Part model, mm, in its own coordinate system. A direction names the side the tool comes from. Round coordinates to 2 decimals unless told otherwise and drop trailing zeros. Write each loop counter-clockwise with the first axis right and the second up, starting at its lowest first coordinate (ties: lowest second). Pieces come first, ordered by that corner, then holes. Notation, with made-up numbers: (76, 26.5) -> (111, 26.5) arc R20 cw to (111, 45.5) -> close; hole circle Ø9 at (49.5, 82). An arc over 180 degrees is marked (long way). Return JSON: item names as keys, results as strings. Group by question number.
(1) Tool access for faces 1 (the flat face through (4, 4, -7)), 2 (the flat face through (32, 15, -6)), 3 (the cylindrical face through (1.829, 28.145, -4.098)): list every direction of +Z, -Z, +X, -X, +Y, -Y with a clear straight run to the whole face (end or side of a thin tool).
(2) Drill centre lines: L1, parallel to Y at x = 62.25, z = -8.45; L2, parallel to Y at x = 62.25, z = -4.25; L3, parallel to X at y = 2.7, z = -3.25. Where is each one in solid material? Low to high. Write a range as from..to.
(3) Saw through at B-B (y = 15). List the corners of the cut face in (x, z).
(4) Saw through at C-C (z = -8.25). List the corners of the cut face in (x, y).
(5) Saw through at A-A (z = -1.5). List the corners of the cut face in (x, y), plus the area to 3 significant figures.
(6) Saw through at D-D (x = 27). List the corners of the cut face in (y, z), plus the area to 3 significant figures.
(7) Mould opens along Y. For faces 4 (the cylindrical face through (0.9, 29.14, -4.56)), 5 (the cylindrical face through (63.405, 2.221, -3.253)), 6 (the cylindrical face through (2.49, 29.283, -8.014)), 7 (the cylindrical face through (-5.5, 15.1, -7.5)) say: +Y half, -Y half, draft (parallel to the pull), parting line (faces both ways), or undercut.
(8) Drop flat-ended pins along their axis: pin 1 Ø3 at (x, y) = (62.25, 27.3) entering from -Z; pin 2 Ø2 at (y, z) = (10, -3.5) entering from -X; pin 3 Ø0.7 at (y, z) = (20.5, 0.5) entering from -X. Give the stop position or say it passes through.
from build123d import *

# Parameters (mm, degrees)
PAD002_DEPTH    = 9
POCKET002_DEPTH = 6
PAD003_DEPTH    = 0.6
SKETCH007_R     = 2
POCKET003_DEPTH = 2
SKETCH008_R     = 1.25
POCKET004_DEPTH = 10
PAD004_DEPTH    = 3


with BuildPart() as part:
    # Sketch004 → Pad002 (new body)
    with BuildSketch(Plane.XY):
        with BuildLine():
            Line((0, 27), (0, 3))
            ThreePointArc((0, 3), (0.87868, 0.87868), (3, 0))
            Line((3, 0), (62, 0))
            ThreePointArc((62, 0), (64.12132, 0.87868), (65, 3))
            Line((65, 3), (65, 27))
            ThreePointArc((65, 27), (64.12132, 29.12132), (62, 30))
            Line((62, 30), (3, 30))
            ThreePointArc((3, 30), (0.87868, 29.12132), (0, 27))
        make_face()
    extrude(amount=PAD002_DEPTH)

    # Sketch005 → Pocket002 (cut)
    with BuildSketch(Plane.XY.offset(9)):
        with BuildLine():
            Line((1.6, 27), (1.6, 3))
            ThreePointArc((1.6, 3), (2.010051, 2.010051), (3, 1.6))
            Line((3, 1.6), (62, 1.6))
            ThreePointArc((62, 1.6), (62.989949, 2.010051), (63.4, 3))
            Line((63.4, 3), (63.4, 27))
            ThreePointArc((63.4, 27), (62.989949, 27.989949), (62, 28.4))
            Line((62, 28.4), (3, 28.4))
            ThreePointArc((3, 28.4), (2.010051, 27.989949), (1.6, 27))
        make_face()
    extrude(amount=-POCKET002_DEPTH, mode=Mode.SUBTRACT)

    # Sketch006 → Pad003 (join)
    with BuildSketch(Plane.XY.offset(9)):
        with BuildLine():
            Line((1.1, 27), (1.1, 3))
            ThreePointArc((1.1, 3), (1.656497, 1.656497), (3, 1.1))
            Line((3, 1.1), (62, 1.1))
            ThreePointArc((62, 1.1), (63.343503, 1.656497), (63.9, 3))
            Line((63.9, 3), (63.9, 27))
            ThreePointArc((63.9, 27), (63.343503, 28.343503), (62, 28.9))
            Line((62, 28.9), (3, 28.9))
            ThreePointArc((3, 28.9), (1.656497, 28.343503), (1.1, 27))
        make_face()
        with BuildLine():
            Line((1.6, 27), (1.6, 3))
            ThreePointArc((1.6, 3), (2.010051, 2.010051), (3, 1.6))
            Line((3, 1.6), (62, 1.6))
            ThreePointArc((62, 1.6), (62.989949, 2.010051), (63.4, 3))
            Line((63.4, 3), (63.4, 27))
            ThreePointArc((63.4, 27), (62.989949, 27.989949), (62, 28.4))
            Line((62, 28.4), (3, 28.4))
            ThreePointArc((3, 28.4), (2.010051, 27.989949), (1.6, 27))
        make_face(mode=Mode.SUBTRACT)
    extrude(amount=PAD003_DEPTH)

    # Sketch007 → Pocket003 (cut)
    with BuildSketch(Plane.XY):
        with Locations((2.75, 27.3)):
            Circle(SKETCH007_R)
        with Locations((62.25, 27.3)):
            Circle(SKETCH007_R)
        with Locations((62.25, 2.7)):
            Circle(SKETCH007_R)
        with Locations((2.75, 2.7)):
            Circle(SKETCH007_R)
    extrude(amount=POCKET003_DEPTH, mode=Mode.SUBTRACT)

    # Sketch008 → Pocket004 (cut)
    with BuildSketch(Plane.XY):
        with Locations((2.75, 27.3)):
            Circle(SKETCH008_R)
        with Locations((62.25, 27.3)):
            Circle(SKETCH008_R)
        with Locations((2.75, 2.7)):
            Circle(SKETCH008_R)
        with Locations((62.25, 2.7)):
            Circle(SKETCH008_R)
    extrude(amount=POCKET004_DEPTH, mode=Mode.SUBTRACT)

    # Sketch009 → Pad004 (join)
    with BuildSketch(Plane.XY):
        with BuildLine():
            ThreePointArc((0, 20.5), (-5.5, 15), (0, 9.5))
            Line((0, 11.5), (0, 9.5))
            ThreePointArc((0, 18.5), (-3.5, 15), (0, 11.5))
            Line((0, 20.5), (0, 18.5))
        make_face()
    extrude(amount=PAD004_DEPTH)


with BuildPart() as part_1:
    # Body001 placement: moved
    add(part.part.moved(Location((0, 0, -9))))


solid = part_1.part
Computed values:
{
 "1": {"face 1": "-Z", "face 2": "+Z", "face 3": "+Z, -Z"},
 "2": {"L1": "0.01..0.7, 4.7..25.3, 29.3..29.99", "L2": "0.01..1.45, 28.55..29.99", "L3": "0.02..1.5, 63.5..64.98"},
 "3": {"outline": "(-5.5, -9) -> (-3.5, -9) -> (-3.5, -6) -> (-5.5, -6) -> close; (0, -9) -> (65, -9) -> (65, 0) -> (63.9, 0) -> (63.9, 0.6) -> (63.4, 0.6) -> (63.4, -6) -> (1.6, -6) -> (1.6, 0.6) -> (1.1, 0.6) -> (1.1, 0) -> (0, 0) -> close"},
 "4": {"outline": "(0, 3) arc R3 ccw to (3, 0) -> (62, 0) arc R3 ccw to (65, 3) -> (65, 27) arc R3 ccw to (62, 30) -> (3, 30) arc R3 ccw to (0, 27) -> (0, 20.5) arc R5.5 ccw to (0, 9.5) -> close; hole (0, 11.5) -> (0, 18.5) arc R3.5 ccw to start; hole circle Ø4 at (2.75, 2.7); hole circle Ø4 at (2.75, 27.3); hole circle Ø4 at (62.25, 2.7); hole circle Ø4 at (62.25, 27.3)"},
 "5": {"outline": "(0, 3) arc R3 ccw to (3, 0) -> (62, 0) arc R3 ccw to (65, 3) -> (65, 27) arc R3 ccw to (62, 30) -> (3, 30) arc R3 ccw to (0, 27) -> close; hole (1.6, 3.19) arc R1.25 ccw to (3.34, 1.6) -> (61.66, 1.6) arc R1.25 ccw to (63.4, 3.19) -> (63.4, 26.81) arc R1.25 ccw to (61.66, 28.4) -> (3.34, 28.4) arc R1.25 ccw to (1.6, 26.81) -> close", "area": "286 mm2"},
 "6": {"outline": "(0, -9) -> (30, -9) -> (30, 0) -> (28.9, 0) -> (28.9, 0.6) -> (28.4, 0.6) -> (28.4, -6) -> (1.6, -6) -> (1.6, 0.6) -> (1.1, 0.6) -> (1.1, 0) -> (0, 0) -> close", "area": "110 mm2"},
 "7": {"face 4": "+Y half", "face 5": "undercut", "face 6": "undercut", "face 7": "parting line"},
 "8": {"pin 1": "z = -7", "pin 2": "x = 0", "pin 3": "x = 1.1"}
}
